```python
from build123d import *

# Parameters (mm, degrees)
SKETCH1_R                 = 25
SKETCH1_W                 = 25
SKETCH1_H                 = 18
BOSS_EXTRUDE1_DEPTH       = 15
SKETCH2_R                 = 20
SKETCH2_W                 = 29
SKETCH2_H                 = 22
BOSS_EXTRUDE2_DEPTH       = 3
F_4_0MM_DOWEL_HOLE1_D     = 4
F_8_0MM_DOWEL_HOLE1_D     = 8
F_8_0MM_DOWEL_HOLE1_DEPTH = 16
F_8_0MM_DOWEL_HOLE2_D     = 8
FILLET1_R                 = 3


with BuildPart() as part:
    # Sketch1 → Boss-Extrude1 (new body)
    with BuildSketch(Plane.XY):
        Circle(SKETCH1_R)
        Rectangle(SKETCH1_W, SKETCH1_H, mode=Mode.SUBTRACT)
    extrude(amount=BOSS_EXTRUDE1_DEPTH)

    # Sketch2 → Boss-Extrude2 (add)
    with BuildSketch(Plane.XY.offset(15)):
        Circle(SKETCH2_R)
        Rectangle(SKETCH2_W, SKETCH2_H, mode=Mode.SUBTRACT)
    extrude(amount=BOSS_EXTRUDE2_DEPTH)

    # Ø4.0mm Dowel Hole1 (through all)
    with Locations(Plane.XY.offset(18)):
        with Locations((0, -15)):
            Hole(F_4_0MM_DOWEL_HOLE1_D / 2)

    # Ø8.0mm Dowel Hole1
    with Locations(Plane(origin=(0, 9, 0), x_dir=(-1, 0, 0), z_dir=(0, -1, 0))):
        with Locations((0, -7.5)):
            Hole(F_8_0MM_DOWEL_HOLE1_D / 2, depth=F_8_0MM_DOWEL_HOLE1_DEPTH)

    # Ø8.0mm Dowel Hole2 (through all)
    with Locations(Plane(origin=(0, -9, 0), x_dir=(1, 0, 0), z_dir=(0, 1, 0))):
        with Locations((0, -7.5)):
            Hole(F_8_0MM_DOWEL_HOLE2_D / 2)

    # Fillet1
    fillet1_edges = [part.edges().sort_by_distance(p)[0] for p in [
        (14.5, 11, 16.5),
        (-14.5, 11, 16.5),
        (-14.5, -11, 16.5),
        (14.5, -11, 16.5),
        (-12.5, 9, 7.5),
        (-12.5, -9, 7.5),
        (12.5, -9, 7.5),
        (12.5, 9, 7.5),
    ]]
    fillet(fillet1_edges, radius=FILLET1_R)


solid = part.part
```
Source: CAD feature listing. Evaluate the final solid. Frame: model axes, mm. A direction names the side the tool comes from. Coordinates: 2 decimals unless noted, no trailing zeros. Write each loop counter-clockwise with the first axis right and the second up, starting at its lowest first coordinate (ties: lowest second). Pieces come first, ordered by that corner, then holes. Notation, with made-up numbers: M -28.5,49.5 L -9.5,49.5 A20 ccw -9.5,81.5 Z; hole C 87,18.5 d5. An arc over 180 degrees is marked long. Answer as a JSON object with one key per item and string values.
1. Ray query, L1, parallel to Y at x = 0, z = 16.5; L2, parallel to Z at x = 2, y = 18.5; L3, parallel to Z at x = 0, y = -12. Return the intervals inside material, ascending.
Evaluation:
{"L1": "-20 to -17, -13 to -11, 11 to 20", "L2": "0 to 4.04, 10.96 to 18", "L3": "0 to 3.5, 11.5 to 18"}
2. Contact query for flat-ended pins moving along their axis: P1, Ø1.5, axis at x = -2, z = 16.5, coming from the -Y side; P2, Ø3.5, axis at y = -2, z = 6, coming from the +X side; P3, Ø5, axis at x = -16, y = -14, coming from the -Z side; P4, Ø2, axis at x = 17.5, y = 15.5, coming from the +Z side. Output: stop coordinate, or through.
Evaluation:
{"P1": "y = -19.96", "P2": "x = 25", "P3": "z = 0", "P4": "z = 15"}
3. Cut plane B-B on y = 0. Output: boundary loops of the cut face in (x, z), plus the area to 3 significant figures.
Evaluation:
{"outline": "M -25,0 L -12.5,0 L -12.5,15 L -14.5,15 L -14.5,18 L -20,18 L -20,15 L -25,15 Z; M 12.5,0 L 25,0 L 25,15 L 20,15 L 20,18 L 14.5,18 L 14.5,15 L 12.5,15 Z", "area": "408 mm^2"}
4. Draft query along X for faces 1 (the cylindrical face through (-4.336, -19.524, 16.479)), 2 (the flat face through (0, -11, 16)), 3 (the flat face through (1, 12, 18)), 4 (the cylindrical face through (-11.6, -8.14, 7.6)). Return one class per face: released by +X, released by -X, zero draft, split by the parting line, or undercut.
Evaluation:
{"face 1": "split by the parting line", "face 2": "undercut", "face 3": "zero draft", "face 4": "undercut"}
5. Cut plane C-C on z = 13. Output: boundary loops of the cut face in (x, y).
Evaluation:
{"outline": "C 0,0 d50; hole M -12.5,-6 A3 ccw -9.5,-9 L 9.5,-9 A3 ccw 12.5,-6 L 12.5,6 A3 ccw 9.5,9 L -9.5,9 A3 ccw -12.5,6 Z; hole C 0,-15 d4"}
6. Cut plane D-D on y = 15.5. Output: boundary loops of the cut face in (x, z).
Evaluation:
{"outline": "M -19.62,0 L 19.62,0 L 19.62,15 L 12.64,15 L 12.64,18 L -12.64,18 L -12.64,15 L -19.62,15 Z; hole C 0,7.5 d8"}
7. Cut plane A-A on x = 0. State how many separate pieces and enclosed holes the cut face has, plus the area to 3 significant figures.
Evaluation:
{"separate pieces": "6", "enclosed holes": "0", "area": "238 mm^2"}
8. Access query for faces 5 (the cylindrical face through (13.6, -10.14, 16.52)), 6 (the cylindrical face through (3.815, 17.112, 6.299)), 7 (the cylindrical face through (-11.6, 8.14, 7.6)). Directions: +Z, -Z, +X, -X, +Y, -Y. A direction counts if a zero-diameter tool reaches every point of the face in a straight line with its end or side. Return the directions, or none.
Evaluation:
{"face 5": "+Z", "face 6": "+Y, -Y", "face 7": "+Z, -Z"}
